Build history of the part. All positions in model axes, mm. A direction names the side the tool comes from. Round coordinates to 2 decimals unless told otherwise and drop trailing zeros. Loops run counter-clockwise (first coordinate to the right, second up) from the corner with the lowest first, then second, coordinate; pieces in that order, holes last. Notation, with made-up numbers: M 69.25,-19 L 94.25,-19 A17 cw 94.25,5 Z; hole C -38,72 d1. An arc over 180 degrees is marked long. Use one line per item in the form item = value. Start each with the question number.
```python
from build123d import *

# Parameters (mm, degrees)
F0_R     = 50.8
F0_R_2   = 19.05
F1_DEPTH = 177.8
F3_DEPTH = 38.1
F5_DEPTH = 38.1
F6_R     = 19.05
F7_DEPTH = 66.802
F8_R     = 19.05
F9_DEPTH = 106.68


with BuildPart() as f1:
    # F0 (on Front) → F1 (new body)
    with BuildSketch(Plane.XZ):
        Circle(F0_R)
        Circle(F0_R_2, mode=Mode.SUBTRACT)
    extrude(amount=F1_DEPTH)

    # F2 (on face) → F3 (join)
    with BuildSketch(Plane.XZ.offset(177.8)):
        with BuildLine():
            Line((-50.8, 177.8), (-50.8, 0))
            ThreePointArc((-50.8, 0), (0, 50.8), (50.8, 0))
            Line((50.8, 0), (50.8, 177.8))
            ThreePointArc((50.8, 177.8), (0, 228.6), (-50.8, 177.8))
        make_face()
    extrude(amount=-F3_DEPTH)

    # F4 (on face) → F5 (join)
    with BuildSketch(Plane(origin=(0, 0, 0), x_dir=(-1, 0, 0), z_dir=(0, 1, 0))):
        with BuildLine():
            Line((-50.8, 177.8), (-50.8, 0))
            ThreePointArc((-50.8, 0), (0, 50.8), (50.8, 0))
            Line((50.8, 0), (50.8, 177.8))
            ThreePointArc((50.8, 177.8), (0, 228.6), (-50.8, 177.8))
        make_face()
    extrude(amount=-F5_DEPTH)

    # F6 (on face) → F7 (cut)
    with BuildSketch(Plane.XZ.offset(177.8)):
        with Locations((0, 177.8)):
            Circle(F6_R)
    extrude(amount=-F7_DEPTH, mode=Mode.SUBTRACT)

    # F8 (on face) → F9 (cut)
    with BuildSketch(Plane(origin=(0, 0, 0), x_dir=(-1, 0, 0), z_dir=(0, 1, 0))):
        with Locations((0, 177.8)):
            Circle(F8_R)
    extrude(amount=-F9_DEPTH, mode=Mode.SUBTRACT)


solid = f1.part
```
Q1. Saw through at A-A (x = 0). Give the cut face in (y, z).
Q2. Saw through at C-C (y = -14.5). Give the cut face in (x, z), and give its area (3 significant figures).
Q3. Drop flat-ended pins along their axis: P1, Ø1.5, axis at x = 36, y = -83, coming from the -Z side; P2, Ø23, axis at x = 0, z = 177.8, coming from the -Y side; P3, Ø10, axis at y = -88.5, z = 38, coming from the +X side; P4, Ø3, axis at x = -40, y = -22, coming from the +Z side. Give the stop position or say it passes through.
Q4. Wall check: probe 1 along Z at (x, y) = (0, -11); probe 2 along Y at (x, z) = (37, 160.5); probe 3 along X at (y, z) = (-15, 177). Give the ranges that are in metal, low to high.
Q5. Saw through at B-B (z = 58.5). Give the cut face in (x, y), and give its area (3 significant figures).
Q6. Pull direction Y, two halves, no side cores. Call faces 1 (the face through (1, -38.1, 116)), 2 (the face through (-1, -177.8, 91)), 3 (the face through (50.8, -19, 90)): pulls with the +Y half, pulls with the -Y half, needs draft (parallel to the pull), parting line crosses it, or undercut.
Q7. Tool access for faces 4 (the face through (-50.8, -19, 88)), 5 (the face through (23.44, -87.66, -45.07)): list every direction of +Z, -Z, +X, -X, +Y, -Y with a clear straight run to the whole face (end or side of a thin tool).
Q8. Saw through at D-D (x = 14.5). Give the cut face in (y, z).
Filled in:
q1.outline = M -177.8,-50.8 L 0,-50.8 L 0,-19.05 L -177.8,-19.05 Z; M -177.8,19.05 L 0,19.05 L 0,158.75 L -38.1,158.75 L -38.1,50.8 L -139.7,50.8 L -139.7,158.75 L -177.8,158.75 Z; M -177.8,196.85 L -139.7,196.85 L -139.7,228.6 L -177.8,228.6 Z; M -38.1,196.85 L 0,196.85 L 0,228.6 L -38.1,228.6 Z
q2.outline = M -50.8,0 A50.8 ccw 50.8,0 L 50.8,177.8 A50.8 ccw -50.8,177.8 Z; hole C 0,0 d38.1; hole C 0,177.8 d38.1
q2.area = 23,900 mm²
q3.P1 = -36.58
q3.P2 = through
q3.P3 = 38.62
q3.P4 = 210.94
q4.probe_1 = -50.8 to -19.05, 19.05 to 158.75, 196.85 to 228.6
q4.probe_2 = -177.8 to -139.7, -38.1 to 0
q4.probe_3 = -50.8 to -19.03, 19.03 to 50.8
q5.outline = M -50.8,-177.8 L 50.8,-177.8 L 50.8,-139.7 L -50.8,-139.7 Z; M -50.8,-38.1 L 50.8,-38.1 L 50.8,0 L -50.8,0 Z
q5.area = 7,740 mm²
q6.face_1 = undercut
q6.face_2 = pulls with the -Y half
q6.face_3 = needs draft
q7.face_4 = +Z, -Z, -X, +Y, -Y
q7.face_5 = none
q8.outline = M -177.8,-48.69 L 0,-48.69 L 0,-12.36 L -177.8,-12.36 Z; M -177.8,12.36 L 0,12.36 L 0,165.44 L -38.1,165.44 L -38.1,48.69 L -139.7,48.69 L -139.7,165.44 L -177.8,165.44 Z; M -177.8,190.16 L -139.7,190.16 L -139.7,226.49 L -177.8,226.49 Z; M -38.1,190.16 L 0,190.16 L 0,226.49 L -38.1,226.49 Z
